Autodesk Inventor part; units mm, degrees
ref_plane "Work Plane1" through (0, 0, 5.5) normal (0, 0, 1) x (1, 0, 0)
ref_plane "YZ Plane" through (0, 0, 0) normal (1, 0, 0) x (0, 1, 0)
ref_plane "XZ Plane" through (0, 0, 0) normal (0, 1, 0) x (-1, 0, 0)
sketch "Sketch1" plane through (0, 0, 0) normal (0, 0, 1) x (1, 0, 0)
  circle A0 centre (0, 0) radius 18.65
  dimension "d0" = 37.3
ref_plane "Work Plane1" through (0, 0, 5.5) normal (0, 0, 1) x (1, 0, 0)
sketch "Sketch2" plane through (0, 0, 5.5) normal (0, 0, 1) x (1, 0, 0)
  circle A0 centre (0, 0) radius 15.25
  dimension "d2" = 30.5
loft "Loft1" add profiles "Sketch1", "Sketch2"
sketch "Sketch3" plane through (0, 0, 5.5) normal (0, 0, 1) x (1, 0, 0)
  circle A0 centre (0, 0) radius 3
  line L0 (0, 0) -> (0, -3) construction
  line L1 (-1.8, 2.4) -> (1.8, 2.4)
  dimension "d7" = 6
  dimension "d8" = 5.4
extrude "Extrusion1" cut sketch "Sketch3" against normal through all contours A0 L1 picked at (0.3021, 0.4498)
chamfer "Chamfer1" distance 1.5 angle 45 1 edges at (-18.65, 0, 0)
chamfer "Chamfer2" distance 1.5 angle 45 1 edges at (-15.25, 0, 5.5)
sketch "Sketch4" plane through (0, 0, 5.5) normal (0, 0, 1) x (1, 0, 0)
  circle A0 centre (0, 0) radius 7.5
  arc A1 (-1.8, 2.4) -> (1.8, 2.4) centre (0, 0) ccw
  line L0 (-1.8, 2.4) -> (1.8, 2.4)
  dimension "d17" = 15
extrude "Extrusion2" add sketch "Sketch4" along normal blind 7.5
chamfer "Chamfer3" distance 1.5 angle 45 1 edges at (-7.5, 0, 13)
sketch "Sketch5" plane through (0, 0, 5.5) normal (0, 0, 1) x (1, 0, 0)
  circle A0 centre (0, 11.3137) radius 2
  circle A1 centre (-8, 8) radius 2
  circle A2 centre (-8, -8) radius 2
  line L0 (-8, 8) -> (-8, -8) construction
  circle A3 centre (0, 0) radius 17.8613
  line L1 (-17.8613, 0) -> (0, 0) construction
  circle A4 centre (-11.3137, 0) radius 2
  circle A5 centre (0, 0) radius 11.3137 construction
  line L2 (0, 0) -> (0, 17.8613) construction
  circle A6 centre (0, -11.3137) radius 2
  circle A7 centre (0, 0) radius 7.5
  line L3 (0, 0) -> (0, -17.8613) construction
  circle A8 centre (8, 8) radius 2
  circle A9 centre (8, -8) radius 2
  circle A10 centre (11.3137, 0) radius 2
  point P0 (-8, 0)
  dimension "d23" = 4
  dimension "d24" = 16
  dimension "d25" = 16
extrude "Extrusion3" cut sketch "Sketch5" against normal through all contours A0 | A1 | A2 | A4 | A6 | A8 | A9 | A10
properties part number "ShoulderMiterGear" material "Aluminum 6061"
Source: CAD feature listing. Evaluate the final solid. Frame: model axes, mm. A direction names the side the tool comes from. Round coordinates to 2 decimals unless told otherwise and drop trailing zeros. Loops run counter-clockwise (first coordinate to the right, second up) from the corner with the lowest first, then second, coordinate; pieces in that order, holes last. Notation, with made-up numbers: M -25,52.25 L -13,52.25 A16 cw -13,61.25 Z; hole C 42,0 d2. An arc over 180 degrees is marked long. Return JSON: item names as keys, results as strings. Group by question number.
1. Section query C-C on z = 11. Output: boundary loops of the cut face in (x, y).
2. Material intervals for line 1 along X through (y, z) = (-1, 2); line 2 along Y through (x, z) = (7, 4.25); line 3 along Y through (x, z) = (9.5, 2.75), sorted ascending. Write a range as from..to.
3. Section query A-A on x = 0. Output: boundary loops of the cut face in (y, z), and give its area (3 significant figures).
4. Reachability of faces 1 (the face through (6, -6, 5.5)), 2 (the face through (-0.434, -13.266, 2.788)) from +Z, -Z, +X, -X, +Y, -Y: full face, straight path, thin tool, end or side. Return the list, or none.
5. Pin query (flat end, axial travel): pin 1 (12 mm diameter, centred on x = -8, y = 3.5, fed in from -Z); pin 2 (6.5 mm diameter, centred on x = 8, y = -8, fed in from +Z); pin 3 (3 mm diameter, centred on y = 5.5, z = 8, fed in from +X); pin 4 (3 mm diameter, centred on x = -0.5, z = 7.5, fed in from -Y). Return the tip coordinate at first contact, or that it passes through.
6. Section query B-B on z = 2. State how many separate pieces and enclosed holes the cut face has, and give its area (3 significant figures).
7. Mould query, pull axis X, two halves, no side actions, for faces 3 (the face through (0, 2.4, 6)), 4 (the face through (0, 3, 13)), 5 (the face through (-7.493, -0.33, 8.458)), 6 (the face through (-9.474, 9.352, 2.788)). Classes: released by +X, released by -X, zero draft, split by the parting line, or undercut.
Checks:
{
 "1": {"outline": "C 0,0 d15; hole M -1.8,2.4 A3 ccw long 1.8,2.4 Z"},
 "2": {"line 1": "x = -17.38..-13.05, -9.58..-2.83, 2.83..9.58, 13.05..17.38", "line 2": "y = -14.38..-9.73, -6.27..6.27, 9.73..14.38", "line 3": "y = -14.04..-9.32, -6.68..-0.84, 0.84..6.68, 9.32..14.04"},
 "3": {"outline": "M -17.86,1.28 L -17.15,0 L -13.31,0 L -13.31,5.5 L -13.75,5.5 L -16.04,4.22 Z; M -9.31,0 L -3,0 L -3,13 L -6,13 L -7.5,11.5 L -7.5,5.5 L -9.31,5.5 Z; M 2.4,0 L 9.31,0 L 9.31,5.5 L 7.5,5.5 L 7.5,11.5 L 6,13 L 2.4,13 Z; M 13.31,0 L 17.15,0 L 17.86,1.28 L 16.04,4.22 L 13.75,5.5 L 13.31,5.5 Z", "area": "179 mm²"},
 "4": {"face 1": "+Z", "face 2": "+Z, -Z"},
 "5": {"pin 1": "stops at z = 0", "pin 2": "stops at z = 5.5", "pin 3": "stops at x = 6.34", "pin 4": "stops at y = -7.5"},
 "6": {"separate pieces": "1", "enclosed holes": "9", "area": "825 mm²"},
 "7": {"face 3": "undercut", "face 4": "zero draft", "face 5": "split by the parting line", "face 6": "undercut"}
}
